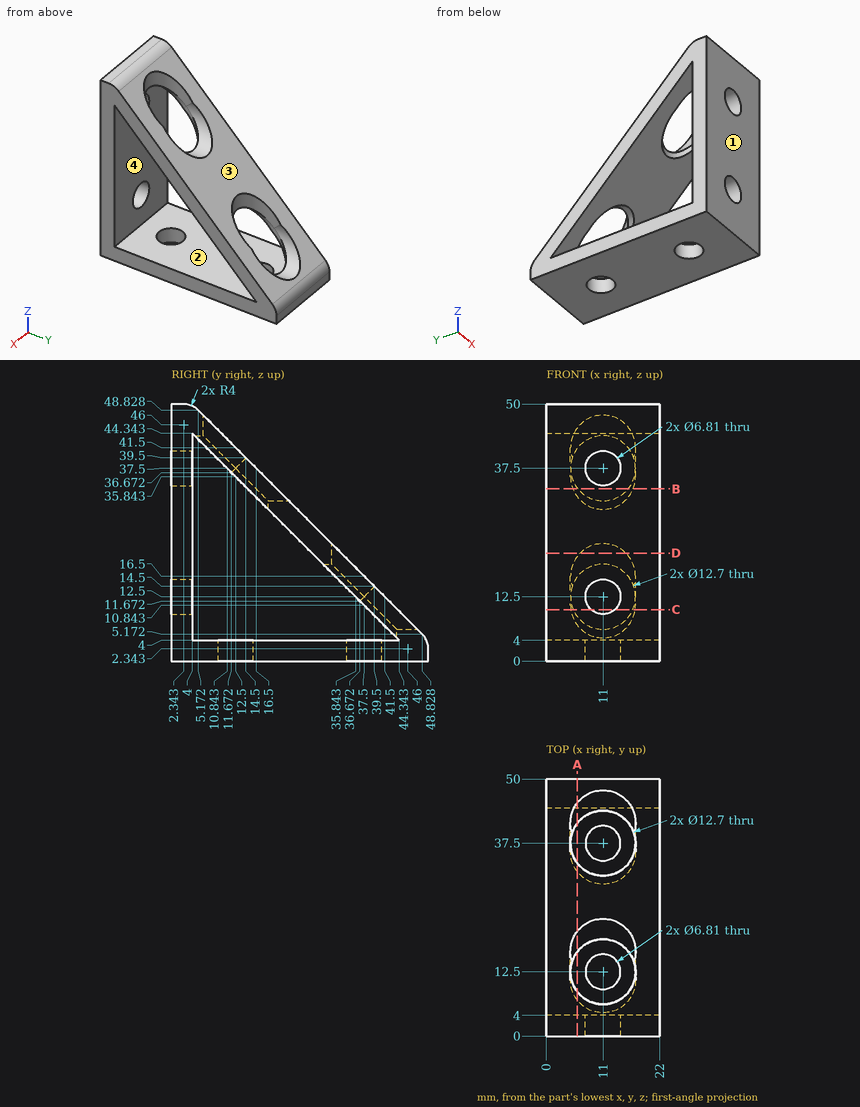
The drawing under review shows one solid part. Ordinate dimensions are in mm from its lowest x, y, z. Give positions to 0.01 mm unless a question says otherwise; leave off trailing zeros. Order: outer loops, then holes, each group sorted by start corner. A loop starts at its lowest first (then second) coordinate and runs counter-clockwise, first axis right, second up. Notation, with made-up numbers: M 82.25,-33.75 L 140.25,-33.75 A25 ccw 140.25,-5.75 Z; hole C -7.5,18.25 d9. An arc over 180 degrees is marked long. Answer in a Markdown table with one row per item. Add a question column.
1. Add section D-D on z = 21. State the section outline as (x, y) points, plus the area to 3 significant figures.
2. Mouldability with a two-part tool opening along Y and no side actions: class the marked faces 1, 2, 3 and 4 as released by +Y, released by -Y, zero draft, split by the parting line, or undercut.
3. Add section A-A on x = 6. State the section outline as (y, z) points (1 decimal).
4. Add section B-B on z = 33.5. State the section outline as (x, y) points.
5. Add section C-C on z = 10. State the section outline as (x, y) points, plus the area to 3 significant figures.
6. To check wall thickness, follow line 1 along Z through (x, y) = (13.5, 9); line 2 along Z through (x, y) = (6.5, 18) (1 decimal). State the ranges of each line that lie inside material, in increasing order.
7. For pin 1 Ø6 at (y, z) = (15, 41.5) entering from +X; pin 2 Ø1.5 at (x, z) = (10.5, 11) entering from +Y; pin 3 Ø7.5 at (x, z) = (11, 12.5) entering from +Y; pin 4 Ø11 at (x, z) = (13.5, 31.5) entering from +Y, all flat-tipped, find the tip position at first contact; note any pin that passes through.
The answers:
| question | item | result |
|---|---|---|
| 1 | outline | M 0,0 L 22,0 L 22,4 L 0,4 Z; M 0,27.34 L 22,27.34 L 22,33 L 15.48,33 A6.35 cw 6.52,33 L 0,33 Z |
| 1 | area | 201 mm2 |
| 2 | face 1 | released by -Y |
| 2 | face 2 | undercut |
| 2 | face 3 | released by +Y |
| 2 | face 4 | undercut |
| 3 | outline | M 0,0 L 50,0 L 50,2.3 A4 ccw 48.8,5.2 L 45.4,8.6 L 41.4,8.6 L 41.4,6.9 L 44.3,4 L 4,4 L 4,44.3 L 6.9,41.4 L 8.6,41.4 L 8.6,45.4 L 5.2,48.8 A4 ccw 2.3,50 L 0,50 Z; M 16.4,31.9 L 31.9,16.4 L 33.6,16.4 L 33.6,20.4 L 20.4,33.6 L 16.4,33.6 Z |
| 4 | outline | M 0,0 L 22,0 L 22,4 L 0,4 Z; M 0,14.84 L 5.1,14.84 A6.35 cw 6.07,16.5 L 6.07,20.5 L 0,20.5 Z; M 15.93,16.5 A6.35 cw 16.9,14.84 L 22,14.84 L 22,20.5 L 15.93,20.5 Z |
| 5 | outline | M 0,0 L 8.69,0 L 8.69,4 L 0,4 Z; M 0,38.34 L 4.71,38.34 A6.35 cw 5.16,40 L 5.16,44 L 0,44 Z; M 13.31,0 L 22,0 L 22,4 L 13.31,4 Z; M 16.84,40 A6.35 cw 17.29,38.34 L 22,38.34 L 22,44 L 16.84,44 Z |
| 5 | area | 127 mm2 |
| 6 | line 1 | 0 to 4 |
| 6 | line 2 | 0 to 4, 30.3 to 33 |
| 7 | pin 1 | x = 22 |
| 7 | pin 2 | through |
| 7 | pin 3 | y = 4 |
| 7 | pin 4 | y = 28 |
